Read the model definition and answer for the solid it produces. Units are mm, in the model's axes. A direction names the side the tool comes from. Coordinates: 2 decimals unless noted, no trailing zeros. Loops run counter-clockwise (first coordinate to the right, second up) from the corner with the lowest first, then second, coordinate; pieces in that order, holes last.
from build123d import *

# Parameters (mm, degrees)
SKETCH1_R           = 1.4
BOSS_EXTRUDE1_DEPTH = 3


with BuildPart() as part:
    # Sketch1 → Boss-Extrude1 (new body)
    with BuildSketch(Plane(origin=(0, 0, 0), x_dir=(1, 0, 0), z_dir=(0, 1, 0))):
        with BuildLine():
            Line((66.715956662, -50.018199395), (23.228889619, -6.531132352))
            ThreePointArc((23.228889619, -6.531132352), (16.157821807, -6.531132352), (16.157821807, -13.602200164))
            Line((16.157821807, -13.602200164), (59.64488885, -57.089267207))
            ThreePointArc((59.64488885, -57.089267207), (59.937782069, -57.796373988), (59.64488885, -58.503480769))
            Line((59.64488885, -58.503480769), (53.63448121, -64.513888409))
            ThreePointArc((53.63448121, -64.513888409), (52.755801554, -66.635208753), (53.63448121, -68.756529097))
            Line((53.63448121, -68.756529097), (59.998442241, -75.120490127))
            ThreePointArc((59.998442241, -75.120490127), (62.119762584, -75.999169784), (64.241082928, -75.120490127))
            Line((64.241082928, -75.120490127), (70.251490568, -69.110082487))
            ThreePointArc((70.251490568, -69.110082487), (70.958597349, -68.817189268), (71.665704131, -69.110082487))
            Line((71.665704131, -69.110082487), (98.535761816, -95.980140172))
            ThreePointArc((98.535761816, -95.980140172), (99.242868597, -96.273033391), (99.949975378, -95.980140172))
            Line((99.949975378, -95.980140172), (105.606829627, -90.323285923))
            ThreePointArc((105.606829627, -90.323285923), (105.899722846, -89.616179142), (105.606829627, -88.90907236))
            Line((105.606829627, -88.90907236), (78.736771942, -62.039014675))
            ThreePointArc((78.736771942, -62.039014675), (78.443878724, -61.331907894), (78.736771942, -60.624801113))
            Line((78.736771942, -60.624801113), (84.747179582, -54.614393473))
            ThreePointArc((84.747179582, -54.614393473), (85.625859239, -52.493073129), (84.747179582, -50.371752786))
            Line((84.747179582, -50.371752786), (78.383218552, -44.007791755))
            ThreePointArc((78.383218552, -44.007791755), (76.261898208, -43.129112099), (74.140577865, -44.007791755))
            Line((74.140577865, -44.007791755), (68.130170225, -50.018199395))
            ThreePointArc((68.130170225, -50.018199395), (67.423063443, -50.311092614), (66.715956662, -50.018199395))
        make_face()
        with Locations((19.693355713, -10.066666258)):
            Circle(SKETCH1_R, mode=Mode.SUBTRACT)
        with BuildLine():
            Line((82.625859239, -70.87784944), (100.303528769, -88.55551897))
            ThreePointArc((100.303528769, -88.55551897), (100.303528769, -90.676839313), (98.182208425, -90.676839313))
            Line((98.182208425, -90.676839313), (80.504538895, -72.999169784))
            ThreePointArc((80.504538895, -72.999169784), (80.504538895, -70.87784944), (82.625859239, -70.87784944))
        make_face(mode=Mode.SUBTRACT)
        with BuildLine():
            Line((59.998442241, -65.220995191), (74.847684646, -50.371752786))
            ThreePointArc((74.847684646, -50.371752786), (78.383218552, -50.371752786), (78.383218552, -53.907286692))
            Line((78.383218552, -53.907286692), (63.533976147, -68.756529097))
            ThreePointArc((63.533976147, -68.756529097), (59.998442241, -68.756529097), (59.998442241, -65.220995191))
        make_face(mode=Mode.SUBTRACT)
        with BuildLine():
            Line((27.825083697, -16.077073898), (57.877121897, -46.129112099))
            ThreePointArc((57.877121897, -46.129112099), (57.877121897, -48.250432442), (55.755801554, -48.250432442))
            Line((55.755801554, -48.250432442), (25.703763353, -18.198394242))
            ThreePointArc((25.703763353, -18.198394242), (25.703763353, -16.077073898), (27.825083697, -16.077073898))
        make_face(mode=Mode.SUBTRACT)
    extrude(amount=BOSS_EXTRUDE1_DEPTH)


solid = part.part
Q1. Determine the mould class of faces 4 (the face through (60, 0, 50)), 5 (the face through (37.597, 1.479, 35.041)), 6 (the face through (76.29, 1.48, 43.13)) for opening direction X: +X half, -X half, draft (parallel to the pull), parting line (faces both ways), or undercut.
Findings below:
face 4: draft
face 5: -X half
face 6: undercut
Q2. A cutting plane is placed at C-C (y = 1.5). Count the separate pieces of the cut face and the enclosed holes in it, then the cut area to 3 significant figures.
Findings below:
separate pieces: 1
enclosed holes: 4
area: 1,230 mm2
Q3. Straight lines are drawn through the part: probe 1 along X at (y, z) = (1.5, 73); probe 2 along X at (y, z) = (2.3, 61); probe 3 along Z at (x, y) = (41, 1.3). For each, find the intervals that lie inside material, in ascending order.
Findings below:
probe 1: x = 57.88 to 66.36, 75.56 to 80.51, 84.75 to 89.7
probe 2: x = 57.15 to 64.22, 71.29 to 78.5
probe 3: z = 24.3 to 29.25, 33.49 to 38.44
Q4. A cutting plane is placed at A-A (z = 35.5). Give the vertices of the cut face in (x, y).
Findings below:
outline: (38.06, 0) - (43.01, 0) - (43.01, 3) - (38.06, 3) - close; (47.25, 0) - (52.2, 0) - (52.2, 3) - (47.25, 3) - close
Q5. Which of the six approach directions +Z, -Z, +X, -X, +Y, -Y give full straight-line access (tool end or side, diameter ignored) to faces 1 (the face through (52.756, 1.479, 66.602)), 2 (the face through (81.7, 1.48, 57.66)), 3 (the face through (67.32, 1.48, 57.9))?
Findings below:
face 1: -X, +Y, -Y
face 2: +X, +Y, -Y
face 3: +Y, -Y
Q6. Flat-ended cylindrical pins translate along their axes: pin 1 Ø1 at (x, y) = (40, 1.5) entering from -Z; pin 2 Ø4.5 at (x, z) = (19.69, 10.07) entering from +Y. Find the tip coordinate at first contact, or state that the pin passes through.
Findings below:
pin 1: stops at z = 22.8
pin 2: stops at y = 3
Q7. A cutting plane is placed at B-B (x = 35). Give the vertices of the cut face in (y, z), then the cut area to 3 significant figures.
Findings below:
outline: (0, 18.3) - (3, 18.3) - (3, 23.25) - (0, 23.25) - close; (0, 27.49) - (3, 27.49) - (3, 32.44) - (0, 32.44) - close
area: 29.7 mm2
